Can you work these out from the model? Positions are in its coordinate system, mm. Face numbers are marked on the shaded views. A direction names the side the tool comes from. Coordinates: 2 decimals unless noted, no trailing zeros. Write each loop counter-clockwise with the first axis right and the second up, starting at its lowest first coordinate (ties: lowest second). Pieces come first, ordered by that corner, then holes. Notation, with made-up numbers: (-23, 13.25) -> (2, 13.25) arc R25 cw to (2, 44.25) -> close; hole circle Ø5 at (0, 22). An arc over 180 degrees is marked (long way). Use one line per item in the form item = value.
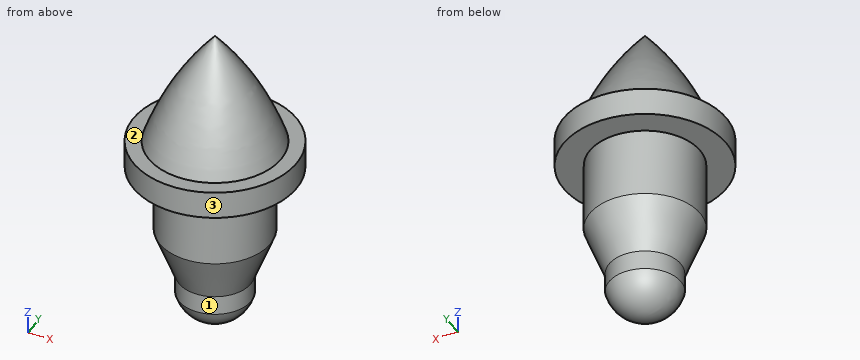
```python
from build123d import *

# Parameters (mm, degrees)
DOME1_FACE_RADIUS = 3.302
DOME1_HEIGHT      = 2.54


# Read off the part's stored shape, not the designer's step: Cut-Revolve-Thin7
with BuildPart() as part:
    # Sketch2 → Revolve1 (revolve)
    with BuildSketch(Plane(origin=(0, 0, 0), x_dir=(0, 0, -1), z_dir=(1, 0, 0)), mode=Mode.PRIVATE) as revolve1_sk:
        Polygon((-8.853714286, 0), (-8.853714286, 7.493), (-6.313714286, 7.493), (-6.313714286, 5.08), (6.386285714, 5.08), (6.386285714, 0), align=None)
    revolve(revolve1_sk.sketch.rotate(Axis((0, 0, 17.845728077), (0, 0, -1)), 90), axis=Axis((0, 0, 17.845728077), (0, 0, -1)))

    # Sketch3 → Revolve2 (revolve)
    with BuildSketch(Plane(origin=(0, 0, 0), x_dir=(0, 0, -1), z_dir=(1, 0, 0))):
        with BuildLine():
            Line((-19.449560173, 0), (-8.853714286, 0))
            Line((-8.853714286, 0), (-8.853714286, 6.085655059))
            add(Edge.make_bspline(
                [(-8.853714286, 6.085655059), (-14.817702659, 4.020762633), (-19.449560173, 0)],
                knots=[0, 0, 0, 1, 1, 1], degree=2))
        make_face()
    revolve(axis=Axis((0, 0, 19.449560173), (0, 0, -1)))

    # Cut-Revolve-Thin7 outline → Cut-Revolve-Thin7 (revolve, cut)
    with BuildSketch(Plane.XZ):
        Polygon((5.08, -0.036285714), (3.302, -4.608285714), (3.302, -6.386285714), (5.08, -6.386285714), align=None)
    revolve(axis=Axis((0, 0, 0), (0, 0, 1)), mode=Mode.SUBTRACT)

    # Dome1: a dome of height H over a round flat face of radius A is a cap of a sphere of radius (A * A + H * H) / (2 * H)
    dome1_r = (DOME1_FACE_RADIUS * DOME1_FACE_RADIUS + DOME1_HEIGHT * DOME1_HEIGHT) / (2 * DOME1_HEIGHT)
    dome1_base = Plane((0, 0, -6.386285714), z_dir=(0, 0, -1))
    with Locations(dome1_base.offset(DOME1_HEIGHT - dome1_r)):
        dome1_ball = Sphere(dome1_r, mode=Mode.PRIVATE)
    add(split(dome1_ball, bisect_by=dome1_base, keep=Keep.TOP, mode=Mode.PRIVATE))


solid = part.part
```
Q1. For the marked faces 1, 2 and 3, which set-ups out of +Z, -Z, +X, -X, +Y, -Y let a thin tool reach every point of the face, with its end or its side?
Return value:
face_1 = -Z
face_2 = +Z
face_3 = +Z, -Z
Q2. Suppose I cut it at A-A (z = -5.75). Write out the boundary of the cut face in (x, y).
Return value:
outline = circle Ø6.6 at (0, 0)
Q3. If I drill on line 1 (Z direction, x = -3.5, y = 5.75); line 2 (X direction, y = -0.75, z = 1); line 3 (X direction, y = -2.25, z = 0.5), over which ranges is the centre line in solid material (lowest first)? Write a range as from..to.
Return value:
line_1 = 6.31..8.85
line_2 = -5.02..5.02
line_3 = -4.55..4.55
Q4. Will these pins go through, and if not, where does the flat tip stop? pin 1 (5 mm diameter, centred on x = 1.5, y = 3.5, fed in from -Z); pin 2 (4 mm diameter, centred on x = 4, z = 9.5, fed in from +Y); pin 3 (1 mm diameter, centred on y = -2, z = 12, fed in from -X).
Return value:
pin_1 = -8.67
pin_2 = 7.19
pin_3 = -4.7
